Check sheet for the modelled part. Datum: model origin and axes. Units: mm. Round coordinates to 2 decimals unless told otherwise and drop trailing zeros. Order: outer loops, then holes, each group sorted by start corner. A loop starts at its lowest first (then second) coordinate and runs counter-clockwise, first axis right, second up. Notation, with made-up numbers: (59.5, 10) -> (108.5, 10) arc R8 cw to (108.5, 25) -> close; hole circle Ø6 at (54.5, -25). An arc over 180 degrees is marked (long way). Answer in a Markdown table with one row per item.
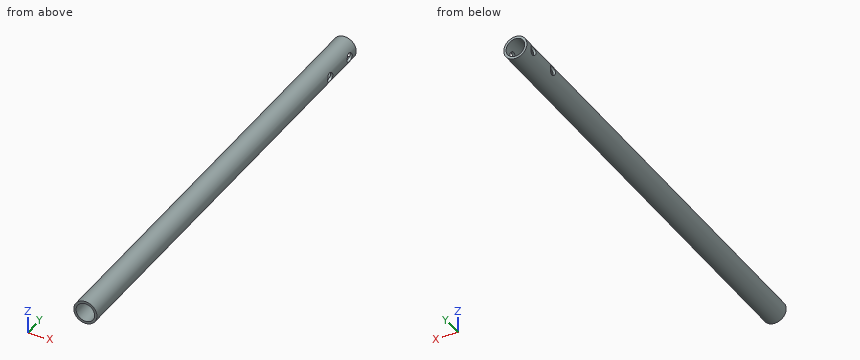
```python
from build123d import *

# Parameters (mm, degrees)
SKETCH_2_R          = 3
SKETCH_2_R_2        = 1.5
EXTRUDE_1_DEPTH     = 200
SKETCH_3_R          = 5
EXTRUDE_2_DEPTH     = 200
SKETCH_4_R          = 4
CUT_EXTRUDE_1_DEPTH = 200
SKETCH_5_R          = 2
CUT_EXTRUDE_5_DEPTH = 100


with BuildPart() as part:
    # 草图2 → 凸台-拉伸1 (new body)
    with BuildSketch(Plane(origin=(0, 0, 0), x_dir=(1, 0, 0), z_dir=(0, 1, 0))):
        with Locations(Location((0, 0, 0), (0, 0, 270))):
            Circle(SKETCH_2_R)
        with Locations(Location((0, 0, 0), (0, 0, 270))):
            Circle(SKETCH_2_R_2, mode=Mode.SUBTRACT)
    extrude(amount=EXTRUDE_1_DEPTH)

    # 草图3 → 凸台-拉伸2 (add)
    with BuildSketch(Plane(origin=(0, 200, 0), x_dir=(1, 0, 0), z_dir=(0, 1, 0))):
        with Locations(Location((0, 0, 0), (0, 0, 270))):
            Circle(SKETCH_3_R)
    extrude(amount=-EXTRUDE_2_DEPTH)

    # 草图4 → 切除-拉伸1 (cut)
    with BuildSketch(Plane(origin=(0, 200, 0), x_dir=(1, 0, 0), z_dir=(0, 1, 0))):
        with Locations(Location((0, 0, 0), (0, 0, 270))):
            Circle(SKETCH_4_R)
    extrude(amount=-CUT_EXTRUDE_1_DEPTH, mode=Mode.SUBTRACT)

    # 草图5 → 切除-拉伸5 (cut, symmetric)
    with BuildSketch(Plane(origin=(0, 0, 0), x_dir=(0, 0, -1), z_dir=(1, 0, 0))):
        with Locations((0, 195)):
            Circle(SKETCH_5_R)
        with Locations((0, 180)):
            Circle(SKETCH_5_R)
    extrude(amount=CUT_EXTRUDE_5_DEPTH, both=True, mode=Mode.SUBTRACT)


solid = part.part
```
(1) Scan lines: probe 1 along Y at (x, z) = (4.65, 0); probe 2 along X at (y, z) = (108.5, 0); probe 3 along X at (y, z) = (84, -3.5). Record each from-to range of solid material in increasing order. Write a range as from..to.
Solutions:
| item | result |
|---|---|
| probe 1 | 0..178, 182..193, 197..200 |
| probe 2 | -5..-4, 4..5 |
| probe 3 | -3.57..-1.94, 1.94..3.57 |
(2) Depth check by flat-ended pin: pin 1 Ø3 at (y, z) = (180, 0) entering from +X; pin 2 Ø4.5 at (y, z) = (195, 0) entering from -X. Enter the tip coordinate at first touch or a pass-through.
Solutions:
| item | result |
|---|---|
| pin 1 | through |
| pin 2 | x = -5 |
(3) Section check A-A on z = 0. Record the boundary of the cut face in (x, y).
Solutions:
| item | result |
|---|---|
| outline | (-5, 0) -> (-4, 0) -> (-4, 178) -> (-5, 178) -> close; (-5, 182) -> (-4, 182) -> (-4, 193) -> (-5, 193) -> close; (-5, 197) -> (-4, 197) -> (-4, 200) -> (-5, 200) -> close; (4, 0) -> (5, 0) -> (5, 178) -> (4, 178) -> close; (4, 182) -> (5, 182) -> (5, 193) -> (4, 193) -> close; (4, 197) -> (5, 197) -> (5, 200) -> (4, 200) -> close |
(4) Section check C-C on y = 180. Record the boundary of the cut face in (x, z).
Solutions:
| item | result |
|---|---|
| outline | (-4.58, -2) arc R5 ccw to (4.58, -2) -> (3.46, -2) arc R4 cw to (-3.46, -2) -> close; (-4.58, 2) -> (-3.46, 2) arc R4 cw to (3.46, 2) -> (4.58, 2) arc R5 ccw to start |
(5) Section check D-D on y = 146. Record the boundary of the cut face in (x, z).
Solutions:
| item | result |
|---|---|
| outline | circle Ø10 at (0, 0); hole circle Ø8 at (0, 0) |
(6) Section check B-B on x = 0. Record the boundary of the cut face in (y, z), plus the area to 3 significant figures.
Solutions:
| item | result |
|---|---|
| outline | (0, -5) -> (200, -5) -> (200, -4) -> (0, -4) -> close; (0, 4) -> (200, 4) -> (200, 5) -> (0, 5) -> close |
| area | 400 mm^2 |
